```python
from build123d import *

# Parameters (mm, degrees)
F2_R        = 8
F2_R_2      = 6.8
F3_DEPTH    = 30
F4_R        = 6.7244244579
F5_DEPTH    = 2.5
F6_R        = 1
F7_S7_R     = 8
F7_T8_DEPTH = 29


# Not quite as in the source:
# - a fillet or chamfer that OpenCascade refuses, or shapes differently, is made with other operations: its cross-section is extruded or revolved along the edge and cut away or added


with BuildPart() as f1:
    # F0 (on Front) → F1 (revolve)
    with BuildSketch(Plane.XZ):
        Polygon((-20.2, 0), (0, 0), (0, 1.2), (-17.8, 1.2), (-17.8, 10), (-19, 10), (-19, 5), (-20.2, 5), align=None)
    revolve(axis=Axis((0, 0, 6.5113101155), (0, 0, -1)))

    # F2 (on Top) → F3 (join)
    with BuildSketch(Plane.XY):
        with Locations((-9.4, 0)):
            Circle(F2_R)
        with Locations((-9.4, 0)):
            Circle(F2_R_2, mode=Mode.SUBTRACT)
    extrude(amount=F3_DEPTH)

    # F4 (on Top) → F5 (cut, symmetric)
    with BuildSketch(Plane.XY):
        with Locations((-9.4230027523, -0.008787398)):
            Circle(F4_R)
    extrude(amount=F5_DEPTH, both=True, mode=Mode.SUBTRACT)

    # F6
    f6_edges = [f1.edges().sort_by_distance(p)[0] for p in [
        (20.2, 0, 0),
        (-16.147427, -0.008787, 0),
    ]]
    fillet(f6_edges, radius=F6_R)

    # F7: fillet of radius 2 on 2 edges, made by hand

    # F7_s1 → F7_t2 (revolve)
    with BuildSketch(Plane.XZ):
        with BuildLine():
            ThreePointArc((-1.4, 3.2), (-0.8142135624, 1.7857864376), (0.6, 1.2))
            Line((0.6, 1.2), (-1.4, 1.2))
            Line((-1.4, 1.2), (-1.4, 3.2))
        make_face()
    revolve(axis=Axis((-9.4, 0, 1.2), (0, 0, -1)))


with BuildPart() as f7_tool4:
    # F7_s5 → F7_t6 (revolve)
    with BuildSketch(Plane.XZ):
        with BuildLine():
            ThreePointArc((-17.8, 3.2), (-17.2142135624, 1.7857864376), (-15.8, 1.2))
            Line((-15.8, 1.2), (-17.8, 1.2))
            Line((-17.8, 1.2), (-17.8, 3.2))
        make_face()
    revolve(axis=Axis((0, 0, 1.2), (0, 0, -1)))

    # F7_s7 → F7_t8 (cut, symmetric)
    with BuildSketch(Plane.XY.offset(2.2)):
        with Locations((-9.4, 0)):
            Circle(F7_S7_R)
    extrude(amount=F7_T8_DEPTH, both=True, mode=Mode.SUBTRACT)


with BuildPart() as f1_1:
    add(f1.part)

    # F7_t3: union F7_tool4
    add(f7_tool4.part)


solid = f1_1.part
```
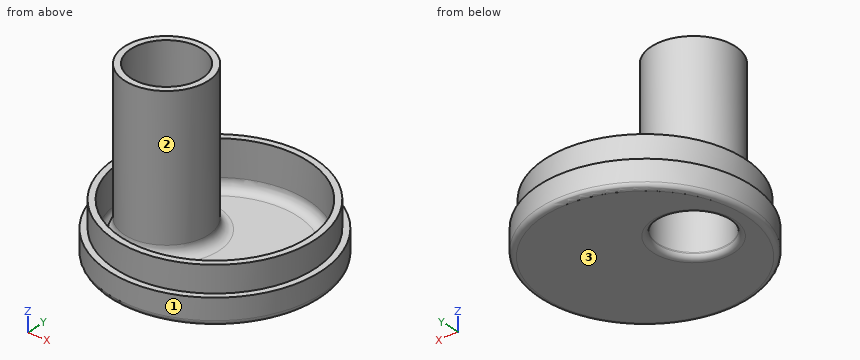
Source: CAD feature listing. Evaluate the final solid. Frame: model axes, mm. Face numbers are marked on the shaded views. Coordinates: 2 decimals unless noted, no trailing zeros. Loops run counter-clockwise (first coordinate to the right, second up) from the corner with the lowest first, then second, coordinate; pieces in that order, holes last. Notation, with made-up numbers: M 47.5,44 L 57.5,44 A19 ccw 57.5,77 Z; hole C 54.25,-28.5 d11. An arc over 180 degrees is marked long. Use CSV: the item, a comma, the result in double quotes.
(1) Line query: line 1 (X direction, y = 0, z = 17.5); line 2 (Y direction, x = -9.4, z = 22); line 3 (Y direction, x = 0, z = 6.5). Output: solid intervals per line, ascending. Write a range as [from, to].
Answers follow:
line 1,"[-17.4, -16.2], [-2.6, -1.4]"
line 2,"[-8, -6.8], [6.8, 8]"
line 3,"[-19, -17.8], [17.8, 19]"
(2) Cut plane A-A on z = 14.5. Return loops of the section in (x, y), and give its area (3 significant figures).
Answers follow:
outline,"C -9.4,0 d16; hole C -9.4,0 d13.6"
area,"55.8 mm²"
(3) Draft query along Y for the marked faces 1, 2 and 3. Return one class per face: pulls with the +Y half, pulls with the -Y half, needs draft (parallel to the pull), parting line crosses it, or undercut.
Answers follow:
face 1,"parting line crosses it"
face 2,"undercut"
face 3,"needs draft"
(4) Contact query for flat-ended pins moving along their axis: pin 1 (10 mm diameter, centred on y = 9.5, z = 25, fed in from +X); pin 2 (22 mm diameter, centred on x = -9.4, y = 0, fed in from -Z); pin 3 (10 mm diameter, centred on y = -7, z = 14, fed in from +X); pin 4 (4 mm diameter, centred on x = -7, y = -2.5, fed in from +Z). Output: stop coordinate, or through.
Answers follow:
pin 1,"x = -2.79"
pin 2,"z = 0"
pin 3,"x = 18.57"
pin 4,"through"
